```python
from build123d import *

# Parameters (mm, degrees)
SKETCH3_W              = 300
SKETCH3_H              = 800
BASE_FLANGE1_DEPTH     = 10
SKETCHED_START         = -168.410340007
SKETCHED_BEND1_DEPTH   = 300
SKETCHED_BEND1_2_DEPTH = 300
BREAK_CORNER1_DEPTH    = 10
BREAK_CORNER1_START    = 9.617841009
BREAK_CORNER1_2_DEPTH  = 10
F_10_0MM_DOWEL_HOLE1_D = 10
F_10_0MM_DOWEL_HOLE2_D = 10
F_10_0MM_DOWEL_HOLE3_D = 10
F_16_0MM_DOWEL_HOLE1_D = 16


# Read off the part's stored shape, not the designer's step: Sketched Bend1, Break-Corner1
# Sheet-metal steps are written as plain solids
with BuildPart() as part:
    # Sketch3 → Base-Flange1 (new body)
    with BuildSketch(Plane(origin=(0, 0, 0), x_dir=(1, 0, 0), z_dir=(0, 1, 0))):
        with Locations((-18.410340007, 84.151074095)):
            Rectangle(SKETCH3_W, SKETCH3_H)
    extrude(amount=BASE_FLANGE1_DEPTH)

    # Sketched Bend1 outline → Sketched Bend1 (cut)
    with BuildSketch(Plane.YZ.offset(SKETCHED_START)):
        with BuildLine():
            Line((10, -484.151074095), (10, 9.643138567))
            ThreePointArc((10, 9.643138567), (2.888569702, 13.027572646), (0, 20.354441009))
            Line((0, 20.354441009), (0, -484.151074095))
            Line((0, -484.151074095), (10, -484.151074095))
        make_face()
    extrude(amount=SKETCHED_BEND1_DEPTH, mode=Mode.SUBTRACT)

    # Sketched Bend1 2 outline → Sketched Bend1 2 (add)
    with BuildSketch(Plane.YZ.offset(SKETCHED_START)):
        with BuildLine():
            Line((10.7366, 9.617841009), (506.231084896, 9.617841009))
            Line((506.231084896, 9.617841009), (506.231084896, 19.617841009))
            Line((506.231084896, 19.617841009), (10.7366, 19.617841009))
            ThreePointArc((10.7366, 19.617841009), (10.215745145, 19.833586154), (10, 20.354441009))
            Line((10, 20.354441009), (10, 9.643138567))
            ThreePointArc((10, 9.643138567), (10.368082861, 9.624167262), (10.7366, 9.617841009))
        make_face()
    extrude(amount=SKETCHED_BEND1_2_DEPTH)

    # Break-Corner1 outline → Break-Corner1 (cut)
    with BuildSketch(Plane(origin=(0, 0, 0), x_dir=(1, 0, 0), z_dir=(0, 1, 0))):
        with BuildLine():
            Line((131.589659993, -315.848925905), (131.589659993, -305.848925905))
            ThreePointArc((131.589659993, -305.848925905), (128.660727805, -312.919993717), (121.589659993, -315.848925905))
            Line((121.589659993, -315.848925905), (131.589659993, -315.848925905))
        make_face()
        with BuildLine():
            Line((-168.410340007, -315.848925905), (-158.410340007, -315.848925905))
            ThreePointArc((-158.410340007, -315.848925905), (-165.481407819, -312.919993717), (-168.410340007, -305.848925905))
            Line((-168.410340007, -305.848925905), (-168.410340007, -315.848925905))
        make_face()
    extrude(amount=BREAK_CORNER1_DEPTH, mode=Mode.SUBTRACT)

    # Break-Corner1 2 outline → Break-Corner1 2 (cut)
    with BuildSketch(Plane.XY.offset(BREAK_CORNER1_START)):
        with BuildLine():
            Line((131.589659993, 506.231084896), (121.589659993, 506.231084896))
            ThreePointArc((121.589659993, 506.231084896), (128.660727805, 503.302152708), (131.589659993, 496.231084896))
            Line((131.589659993, 496.231084896), (131.589659993, 506.231084896))
        make_face()
        with BuildLine():
            ThreePointArc((-168.410340007, 496.231084896), (-165.481407819, 503.302152708), (-158.410340007, 506.231084896))
            Line((-158.410340007, 506.231084896), (-168.410340007, 506.231084896))
            Line((-168.410340007, 506.231084896), (-168.410340007, 496.231084896))
        make_face()
    extrude(amount=BREAK_CORNER1_2_DEPTH, mode=Mode.SUBTRACT)

    # Ø10.0mm Dowel Hole1 (through all)
    with Locations(Plane.XY.offset(19.617841009)):
        with Locations((-13.684653237, 333.231084896), (-13.684653237, 233.231084896), (-13.684653237, 133.231084896)):
            Hole(F_10_0MM_DOWEL_HOLE1_D / 2)

    # Ø10.0mm Dowel Hole2 (through all)
    with Locations(Plane(origin=(0, 10, 0), x_dir=(1, 0, 0), z_dir=(0, 1, 0))):
        with Locations((-13.042040007, -86.690456915), (-13.042040007, -159.007394895)):
            Hole(F_10_0MM_DOWEL_HOLE2_D / 2)

    # Ø10.0mm Dowel Hole3 (through all)
    with Locations(Plane.XY.offset(19.617841009)):
        with Locations((85.847745748, 471.172292647), (85.847745748, 413.289877144), (-122.668425763, 413.289877144), (-122.668425763, 471.172292647)):
            Hole(F_10_0MM_DOWEL_HOLE3_D / 2)

    # Ø16.0mm Dowel Hole1 (through all)
    with Locations(Plane(origin=(0, 10, 0), x_dir=(1, 0, 0), z_dir=(0, 1, 0))):
        with Locations((-128.305039397, -66.908688048), (91.484359382, -66.908688048), (91.484359382, -268.558078866), (-128.305039397, -268.558078866)):
            Hole(F_16_0MM_DOWEL_HOLE1_D / 2)


solid = part.part
```
Check sheet for the modelled part. Datum: model origin and axes. Units: mm. A direction names the side the tool comes from. Round coordinates to 2 decimals unless told otherwise and drop trailing zeros. Write each loop counter-clockwise with the first axis right and the second up, starting at its lowest first coordinate (ties: lowest second). Pieces come first, ordered by that corner, then holes. Notation, with made-up numbers: M 52,-21.75 L 66,-21.75 A21 cw 66,-7.75 Z; hole C 21,54.25 d8. An arc over 180 degrees is marked long. Write item = value, one per line. Start each with the question number.
1. Section check A-A, the plane x = -100.5. Record the cut outline in (y, z), then the cut area to 3 significant figures.
2. Section check B-B, the plane z = 234.5. Record the cut outline in (x, y).
3. Scan lines: line 1 (Y direction, x = 61, z = 108); line 2 (Z direction, x = 22.5, y = 200.5). Record each from-to range of solid material in increasing order. Write a range as [from, to].
4. Release check for a two-part mould opening along X. For faces 3 (the cylindrical face through (89.82, 410.25, 14.55)), 4 (the cylindrical face through (-165.56, 503.22, 14.55)), 5 (the flat face through (-20, 506.231, 15)) record: pulls with the +X half, pulls with the -X half, needs draft (parallel to the pull), parting line crosses it, or undercut.
5. Gauge pin test, flat ends, axial feed: pin 1 (11.5 mm diameter, centred on x = 85.85, y = 413.29, fed in from +Z); pin 2 (21 mm diameter, centred on x = 91.48, z = 66.91, fed in from +Y); pin 3 (2 mm diameter, centred on x = -60, z = 90, fed in from -Y). Record the tip position at first contact, or that the pin passes through.
6. Section check C-C, the plane y = 47. Record the cut outline in (x, z), then the cut area to 3 significant figures.
7. Tool access check on faces 1 (the flat face through (-21, 262, 19.618)), 2 (the flat face through (-21, 255, 9.618)). Record the directions out of +Z, -Z, +X, -X, +Y, -Y that give a thin tool (end or side, any length) a straight path to the whole face; none if there is none.
Results found:
q1.outline = M 0,20.35 A10.74 ccw 10.74,9.62 L 506.23,9.62 L 506.23,19.62 L 10.74,19.62 A0.74 cw 10,20.35 L 10,315.85 L 0,315.85 Z
q1.area = 8,000 mm^2
q2.outline = M -168.41,0 L 131.59,0 L 131.59,10 L -168.41,10 Z
q3.line_1 = [0, 10]
q3.line_2 = [9.62, 19.62]
q4.face_3 = undercut
q4.face_4 = pulls with the -X half
q4.face_5 = needs draft
q5.pin_1 = 19.62
q5.pin_2 = 10
q5.pin_3 = 0
q6.outline = M -168.41,9.62 L 131.59,9.62 L 131.59,19.62 L -168.41,19.62 Z
q6.area = 3,000 mm^2
q7.face_1 = +Z, +X, -X, +Y
q7.face_2 = -Z, +X, -X, +Y, -Y
